For this review, take the finished solid that the model builds, in its own axes (mm). A direction names the side the tool comes from. Round coordinates to 2 decimals unless told otherwise and drop trailing zeros. Loops run counter-clockwise (first coordinate to the right, second up) from the corner with the lowest first, then second, coordinate; pieces in that order, holes last.
1. Consider section B-B on x = 20. State the section outline as (y, z) points.
2. To check wall thickness, follow line 1 along Y through (x, z) = (-15, 4.5); line 2 along X through (y, z) = (1, -4); line 3 along X through (y, z) = (-13, 11.5). State the ranges of each line that lie inside material, in increasing order.
3. Clearance check with flat-ended pins moving along their axes: pin 1 Ø2 at (x, y) = (-19, -11.5) entering from +Z; pin 2 Ø10 at (y, z) = (1, 3) entering from -X; pin 3 Ø5 at (x, y) = (-7.5, 2) entering from -Z; pin 4 Ø8 at (y, z) = (-5.5, -12) entering from -X. State where each tip first meets the part, or that it passes through.
4. Tool access review of faces 4 (the cylindrical face through (-17.34, -7.5, -11.55)), 5 (the cylindrical face through (-12.505, 17.986, 0.22)), 6 (the cylindrical face through (-27.99, -8.11, -5.97)): name each direction out of +Z, -Z, +X, -X, +Y, -Y from which nothing blocks a thin tool from reaching the whole face with its end or side.
5. Draft analysis for pull direction X (two halves, no side actions). For faces 1 (the flat face through (27.5, 0, 0)), 2 (the flat face through (-26.5, -10.7, 14)), 3 (the flat face through (6.5, 14, -0.1)), state which applies: released by +X, released by -X, zero draft, split by the parting line, or undercut.
6. Consider section D-D on y = -12.5. State the section outline as (x, z) points, then the cut area to 3 significant figures.
from build123d import *

# Parameters (mm, degrees)
F1_DEPTH  = 15
F3_DEPTH  = 7
F4_R      = 6.5
F5_SIZE   = 2
F6_W      = 14
F6_H      = 9
F7_DEPTH  = 30.001
F8_R      = 5
F9_R      = 3
F10_DEPTH = 1
F11_R     = 3
F12_DEPTH = 15
F13_R     = 5
F14_DEPTH = 4
F15_SIZE  = 1.99999


# Not quite as in the source:
# - a fillet or chamfer is up to 0.001 mm smaller than in the source, because OpenCascade refuses the exact size
# - a pattern or mirror of a feature is missing from the dataset's text; its kind, count and spacing are read off the source's solid


with BuildPart() as f1:
    # F0 (on Top) → F1 (new body, symmetric)
    with BuildSketch(Plane.XY):
        Polygon((27.5, 15), (5.5, 15), (5.5, 0), (-27.5, 0), (-27.5, -15), (27.5, -15), align=None)
    extrude(amount=F1_DEPTH, both=True)

    # F2 (on face) → F3 (cut)
    with BuildSketch(Plane.XY.offset(15)):
        with BuildLine():
            Line((-25, -15), (-10, -15))
            ThreePointArc((-10, -15), (-17.5, -7.5), (-25, -15))
        make_face()
        with BuildLine():
            ThreePointArc((25, -15), (17.5, -7.5), (10, -15))
            Line((10, -15), (25, -15))
        make_face()
    f3 = extrude(amount=-F3_DEPTH, mode=Mode.SUBTRACT)

    # F3_copies: F3 across plane
    add(f3.mirror(Plane(origin=(0, 0, 0), x_dir=(-1, 0, 0), z_dir=(0, 0, -1))), mode=Mode.SUBTRACT)

    # F4
    f4_edges = [f1.edges().sort_by_distance(p)[0] for p in [
        (-11, 0, 15),
        (-11, 0, -15),
        (5.5, 7.5, 15),
        (5.5, 7.5, -15),
    ]]
    fillet(f4_edges, radius=F4_R)

    # F5
    f5_edges = [f1.edges().sort_by_distance(p)[0] for p in [
        (5.5, 15, 0),
        (-27.5, 0, 0),
    ]]
    chamfer(f5_edges, length=F5_SIZE)

    # F6 (on face) → F7 (cut, through all)
    with BuildSketch(Plane.XY.offset(15)):
        with Locations((19.0077603161, 6.4331619842)):
            Rectangle(F6_W, F6_H)
    extrude(amount=-F7_DEPTH, mode=Mode.SUBTRACT)

    # F8
    f8_edges = [f1.edges().sort_by_distance(p)[0] for p in [
        (19.00776, 1.933162, 15),
        (26.00776, 10.933162, 0),
        (12.00776, 10.933162, 0),
    ]]
    fillet(f8_edges, radius=F8_R)

    # F9 (on face) → F10 (join)
    with BuildSketch(Plane(origin=(-27.5, 0, 0), x_dir=(0, -1, 0), z_dir=(-1, 0, 0))):
        with Locations((6.5, 8.5)):
            Circle(F9_R)
        with Locations((6.5, -8.5)):
            Circle(F9_R)
    extrude(amount=F10_DEPTH)

    # F11 (on face) → F12 (join)
    with BuildSketch(Plane(origin=(0, 0, 0), x_dir=(-1, 0, 0), z_dir=(0, 1, 0))):
        with Locations((17.5, 0)):
            Circle(F11_R)
    extrude(amount=F12_DEPTH)

    # F13 (on face) → F14 (join)
    with BuildSketch(Plane(origin=(0, 15, 0), x_dir=(-1, 0, 0), z_dir=(0, 1, 0))):
        with Locations((17.5, 0)):
            Circle(F13_R)
    extrude(amount=F14_DEPTH)

    # F15 (size 2 in the source; OpenCascade refuses exactly that, so slightly less here)
    f15_edges = [f1.edges().sort_by_distance(p)[0] for p in [
        (-12.5, 15, 0),
    ]]
    chamfer(f15_edges, length=F15_SIZE)


solid = f1.part
Resolved:
1. outline: (-15, -8) - (-7.93, -8) - (-7.93, -15) - (1.93, -15) - (1.93, 10) arc R5 ccw to (-3.07, 15) - (-7.93, 15) - (-7.93, 8) - (-15, 8) - close; (10.93, -15) - (13, -15) - (15, -13) - (15, 13) - (13, 15) - (10.93, 15) - close
2. line 1: y = -15 to 0
2. line 2: x = 5.5 to 27.5
2. line 3: x = -27.5 to -24.73, -10.27 to 10.27, 24.73 to 27.5
3. pin 1: stops at z = 8
3. pin 2: stops at x = -27.5
3. pin 3: stops at z = -11
3. pin 4: stops at x = -28.5
4. face 4: -Z, -Y
4. face 5: +Y
4. face 6: -X
5. face 1: released by +X
5. face 2: released by -X
5. face 3: undercut
6. outline: (-27.5, -13) - (-25.5, -15) - (-24.57, -15) - (-24.57, -8) - (-10.43, -8) - (-10.43, -15) - (10.43, -15) - (10.43, -8) - (24.57, -8) - (24.57, -15) - (27.5, -15) - (27.5, 15) - (24.57, 15) - (24.57, 8) - (10.43, 8) - (10.43, 15) - (-10.43, 15) - (-10.43, 8) - (-24.57, 8) - (-24.57, 15) - (-25.5, 15) - (-27.5, 13) - close
6. area: 1,250 mm2
